```python
from build123d import *

# Parameters (mm, degrees)
SKETCH1_W           = 25.4
SKETCH1_H           = 25.4
SKETCH1_W_2         = 22.225
SKETCH1_H_2         = 22.225
BOSS_EXTRUDE1_DEPTH = 101.6
SKETCH2_R           = 1.984375
CUT_EXTRUDE1_DEPTH  = 26.4


with BuildPart() as part:
    # Sketch1 → Boss-Extrude1 (new body)
    with BuildSketch(Plane.XY):
        Rectangle(SKETCH1_W, SKETCH1_H)
        Rectangle(SKETCH1_W_2, SKETCH1_H_2, mode=Mode.SUBTRACT)
    extrude(amount=BOSS_EXTRUDE1_DEPTH)

    # Sketch2 → Cut-Extrude1 (cut, through all)
    with BuildSketch(Plane(origin=(0, 12.7, 0), x_dir=(1, 0, 0), z_dir=(0, 1, 0))):
        with Locations((0, -88.9)):
            Circle(SKETCH2_R)
        with Locations((0, -63.5)):
            Circle(SKETCH2_R)
        with Locations((0, -38.1)):
            Circle(SKETCH2_R)
        with Locations((0, -12.7)):
            Circle(SKETCH2_R)
        with Locations((0, 12.7)):
            Circle(SKETCH2_R)
        with Locations((0, 38.1)):
            Circle(SKETCH2_R)
        with Locations((0, 63.5)):
            Circle(SKETCH2_R)
        with Locations((0, 88.9)):
            Circle(SKETCH2_R)
        with Locations((0, 114.3)):
            Circle(SKETCH2_R)
        with Locations((0, 139.7)):
            Circle(SKETCH2_R)
        with Locations((0, 165.1)):
            Circle(SKETCH2_R)
        with Locations((0, 190.5)):
            Circle(SKETCH2_R)
    extrude(amount=-CUT_EXTRUDE1_DEPTH, mode=Mode.SUBTRACT)


solid = part.part
```
Build history of the part. All positions in model axes, mm. A direction names the side the tool comes from. Give positions to 0.01 mm unless a question says otherwise; leave off trailing zeros. Loops run counter-clockwise (first coordinate to the right, second up) from the corner with the lowest first, then second, coordinate; pieces in that order, holes last.
Item 1: Flat gauge pin, fed straight in: pin 1 (3.5 mm diameter, centred on x = 0, z = 88.9, fed in from -Y). Where does the tip first touch, or does it go through?
Answers follow:
pin 1: passes through
Item 2: Pull direction Z, two halves, no side cores. Call faces 1 (the face through (-0.43, -11.895, 14.637)), 2 (the face through (-12.7, 0, 50)), 3 (the face through (1.07, 11.92, 87.23)), 4 (the face through (-11.3, 0.1, 101.6)): released by +Z, released by -Z, zero draft, split by the parting line, or undercut.
Answers follow:
face 1: undercut
face 2: zero draft
face 3: undercut
face 4: released by +Z
Item 3: Slice it at C-C, the plane z = 38.1. List the corners of the cut face in (x, y), and give its area (3 significant figures).
Answers follow:
outline: (-12.7, -12.7) - (-1.98, -12.7) - (-1.98, -11.11) - (-11.11, -11.11) - (-11.11, 11.11) - (-1.98, 11.11) - (-1.98, 12.7) - (-12.7, 12.7) - close; (1.98, -12.7) - (12.7, -12.7) - (12.7, 12.7) - (1.98, 12.7) - (1.98, 11.11) - (11.11, 11.11) - (11.11, -11.11) - (1.98, -11.11) - close
area: 139 mm2
Item 4: Slice it at D-D, the plane x = 0. Give the number of separate pieces and of enclosed holes in the cut face, and give its area (3 significant figures).
Answers follow:
separate pieces: 10
enclosed holes: 0
area: 272 mm2
Item 5: Which spindle directions (+Z, -Z, +X, -X, +Y, -Y) get a long thin tool onto all of the face, cutting with end or side? Do faces 5 (the face through (0, 12.7, 50)), 6 (the face through (11.112, 0, 50)). Say none if no direction does.
Answers follow:
face 5: +Z, -Z, +X, -X, +Y
face 6: +Z, -Z
Item 6: Slice it at A-A, the plane x = 5. List the corners of the cut face in (y, z).
Answers follow:
outline: (-12.7, 0) - (-11.11, 0) - (-11.11, 101.6) - (-12.7, 101.6) - close; (11.11, 0) - (12.7, 0) - (12.7, 101.6) - (11.11, 101.6) - close
Item 7: Drill centre lines: line 1 (Z direction, x = 0, y = 12.25); line 2 (X direction, y = 3.25, z = 41.5). Where is each one in solid material? Low to high.
Answers follow:
line 1: z = 0 to 10.72, 14.68 to 36.12, 40.08 to 61.52, 65.48 to 86.92, 90.88 to 101.6
line 2: x = -12.7 to -11.11, 11.11 to 12.7
